```python
from build123d import *

# Parameters (mm, degrees)
F0_R     = 3
F1_DEPTH = 1.5


with BuildPart() as f1:
    # F0 (on Front) → F1 (new body, symmetric)
    with BuildSketch(Plane.XZ):
        with BuildLine():
            ThreePointArc((483.7124742394, 240.4259464291), (475.4570998666, 251.3503928024), (462.4081345934, 255.5))
            Line((462.4081345934, 255.5), (-465, 255.5))
            ThreePointArc((-465, 255.5), (-479.1421356237, 249.6421356237), (-485, 235.5))
            Line((-485, 235.5), (-485, -215.5))
            ThreePointArc((-485, -215.5), (-473.2842712475, -243.7842712475), (-445, -255.5))
            Line((-445, -255.5), (0, -255.5))
            Line((0, -255.5), (435, -255.5))
            ThreePointArc((435, -255.5), (463.2842712475, -243.7842712475), (475, -215.5))
            Line((475, -215.5), (475, -81.5))
            Line((475, -81.5), (475, -76.5))
            ThreePointArc((475, -76.5), (476.4644660941, -72.9644660941), (480, -71.5))
            ThreePointArc((480, -71.5), (483.5355339059, -70.0355339059), (485, -66.5))
            Line((485, -66.5), (485, -61.5))
            Line((485, -61.5), (485, -1.5))
            Line((485, -1.5), (462.8157010189, -1.5))
            Line((462.8157010189, -1.5), (403.7124742394, -1.5))
            ThreePointArc((403.7124742394, -1.5), (393.1058725216, 2.8933982822), (388.7124742394, 13.5))
            Line((388.7124742394, 13.5), (388.7124742394, 167.5))
            ThreePointArc((388.7124742394, 167.5), (393.1058725216, 178.1066017178), (403.7124742394, 182.5))
            Line((403.7124742394, 182.5), (483.7124742394, 182.5))
            Line((483.7124742394, 182.5), (483.7124742394, 240.4259464291))
        make_face()
        with Locations((-470, -205.5)):
            Circle(F0_R, mode=Mode.SUBTRACT)
        with Locations((-410, -215.5)):
            Circle(F0_R, mode=Mode.SUBTRACT)
        with Locations((-100, -240.5)):
            Circle(F0_R, mode=Mode.SUBTRACT)
        with Locations((-470, -19.5)):
            Circle(F0_R, mode=Mode.SUBTRACT)
        with Locations((150, -240.5)):
            Circle(F0_R, mode=Mode.SUBTRACT)
        with Locations((400, -240.5)):
            Circle(F0_R, mode=Mode.SUBTRACT)
        with Locations((450, -180.5)):
            Circle(F0_R, mode=Mode.SUBTRACT)
        with Locations((450.0357970595, -16.4979236722)):
            Circle(F0_R, mode=Mode.SUBTRACT)
        with Locations((-470, 160.5)):
            Circle(F0_R, mode=Mode.SUBTRACT)
        with Locations((-400, 225.5)):
            Circle(F0_R, mode=Mode.SUBTRACT)
        with Locations((-200, 225.5)):
            Circle(F0_R, mode=Mode.SUBTRACT)
        with BuildLine():
            Line((112, 116.5), (112, 150.5))
            ThreePointArc((112, 150.5), (114.9289321881, 157.5710678119), (122, 160.5))
            Line((122, 160.5), (191, 160.5))
            ThreePointArc((191, 160.5), (198.0710678119, 157.5710678119), (201, 150.5))
            Line((201, 150.5), (201, 116.5))
            ThreePointArc((201, 116.5), (198.0710678119, 109.4289321881), (191, 106.5))
            Line((191, 106.5), (122, 106.5))
            ThreePointArc((122, 106.5), (114.9289321881, 109.4289321881), (112, 116.5))
        make_face(mode=Mode.SUBTRACT)
        with Locations((0, 225.5)):
            Circle(F0_R, mode=Mode.SUBTRACT)
        with Locations((200.0356763601, 225.499600172)):
            Circle(F0_R, mode=Mode.SUBTRACT)
        with BuildLine():
            Line((360.7124742394, 147.5), (360.7124742394, 168.5))
            ThreePointArc((360.7124742394, 168.5), (361.298260677, 169.9142135624), (362.7124742394, 170.5))
            Line((362.7124742394, 170.5), (373.7124742394, 170.5))
            ThreePointArc((373.7124742394, 170.5), (375.1266878018, 169.9142135624), (375.7124742394, 168.5))
            Line((375.7124742394, 168.5), (375.7124742394, 147.5))
            ThreePointArc((375.7124742394, 147.5), (375.1266878018, 146.0857864376), (373.7124742394, 145.5))
            Line((373.7124742394, 145.5), (362.7124742394, 145.5))
            ThreePointArc((362.7124742394, 145.5), (361.298260677, 146.0857864376), (360.7124742394, 147.5))
        make_face(mode=Mode.SUBTRACT)
        with Locations((448.759393394, 215.4916015863)):
            Circle(F0_R, mode=Mode.SUBTRACT)
        with Locations((399.9695941806, 225.4816529751)):
            Circle(F0_R, mode=Mode.SUBTRACT)
    extrude(amount=F1_DEPTH, both=True)


solid = f1.part
```
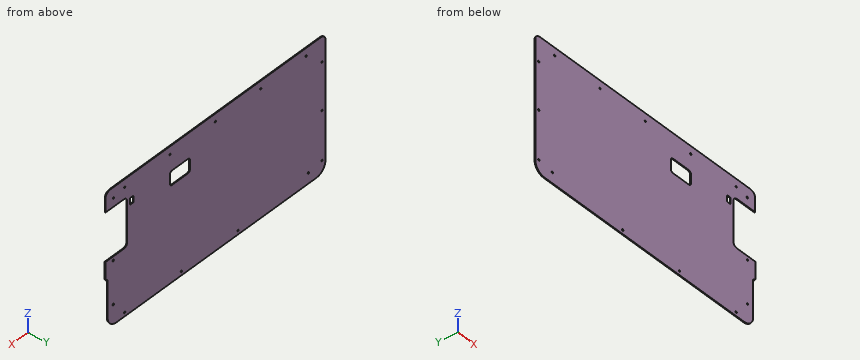
The listing builds one solid part. Answer for the finished solid, in the listing's coordinates (mm). Give positions to 0.01 mm unless a question says otherwise; leave off trailing zeros. Order: outer loops, then holes, each group sorted by start corner. A loop starts at its lowest first (then second) coordinate and runs counter-clockwise, first axis right, second up. Notation, with made-up numbers: (85.5, 77.5) - (94.5, 77.5) arc R7 ccw to (94.5, 86.5) - close; hole circle Ø3 at (3.25, 16.25). An arc over 180 degrees is marked (long way). Use one line per item in the form item = value. Start each with the question number.
(1) A cutting plane is placed at A-A, the plane z = 127. Write down the section's boundary in (x, y), then the cut area to 3 significant figures.
(2) A flat-ended cylindrical pin translates along its axis: pin 1 Ø1.5 at (y, z) = (0.5, 135) entering from +X. Find the tip coordinate at first contact, or state that the pin passes through.
(3) A cutting plane is placed at B-B, the plane y = 0. State how many separate pieces and enclosed holes the cut face has, then the cut area to 3 significant figures.
(4) Consider line 1 (Z direction, x = 0, y = -0.5); line 2 (X direction, y = 0.4, z = 140); line 3 (Z direction, x = -410, y = -0.45). Determine where each line is inside the solid, lowest interval first. Write a range as from..to.
Ans:
q1.outline = (-485, -1.5) - (112, -1.5) - (112, 1.5) - (-485, 1.5) - close; (201, -1.5) - (388.71, -1.5) - (388.71, 1.5) - (201, 1.5) - close
q1.area = 2,350 mm^2
q2.pin_1 = 388.71
q3.separate_pieces = 1
q3.enclosed_holes = 17
q3.area = 470,000 mm^2
q4.line_1 = -255.5..222.5, 228.5..255.5
q4.line_2 = -485..112, 201..388.71
q4.line_3 = -255.5..-218.5, -212.5..255.5
